Autodesk Inventor part; units mm, degrees
ref_plane "YZ Plane" through (0, 0, 0) normal (1, 0, 0) x (0, 1, 0)
ref_plane "XZ Plane" through (0, 0, 0) normal (0, 1, 0) x (-1, 0, 0)
ref_plane "XY Plane" through (0, 0, 0) normal (0, 0, 1) x (1, 0, 0)
sketch "Sketch1" plane through (0, 0, 0) normal (0, 0, 1) x (1, 0, 0)
  line L0 (-7.5, 17.5) -> (7.5, 17.5)
  line L1 (7.5, 17.5) -> (7.5, -17.5)
  line L2 (7.5, -17.5) -> (-7.5, -17.5)
  line L3 (-7.5, -17.5) -> (-7.5, 17.5)
  line L4 (-7.5, 17.5) -> (7.5, -17.5) construction
  line L5 (7.5, 17.5) -> (-7.5, -17.5) construction
  point P0 (0, 0)
  dimension "d0" = 15
  dimension "d1" = 35
extrude "Extrusion1" add sketch "Sketch1" along normal blind 25
sketch "Sketch2" plane through (-7.5, 17.5, 0) normal (0, 1, 0) x (1, 0, 0)
  line L0 (15, -25) -> (0, -25) construction
  line L1 (0, 0) -> (10.4, 0) construction
  line L2 (10.4, 0) -> (10.4, -25) construction
  line L3 (10.4, -25) -> (0, -25) construction
  line L4 (0, -25) -> (0, 0) construction
  line L5 (0, 0) -> (15, 0) construction
  line L6 (5.2, 0) -> (5.2, -25) construction
  line L7 (10.4, -12.5) -> (0, -12.5) construction
  line L8 (0, 0) -> (0, -25) construction
  line L9 (10.4, -4.3) -> (0, -4.3) construction
  line L10 (0, -4.3) -> (0, -20.7) construction
  line L11 (0, -20.7) -> (10.4, -20.7) construction
  line L12 (10.4, -20.7) -> (10.4, -4.3) construction
  line L13 (10.4, -4.3) -> (0, -20.7) construction
  line L14 (0, -4.3) -> (10.4, -20.7) construction
  circle A0 centre (5.2, -9.5) radius 5.2
  circle A1 centre (5.2, -15.5) radius 5.2
  line L15 (10.4, -9.5) -> (0, -9.5)
  line L16 (0, -9.5) -> (0, -15.5)
  line L17 (0, -15.5) -> (10.4, -15.5)
  line L18 (10.4, -15.5) -> (10.4, -9.5)
  line L19 (10.4, -9.5) -> (0, -15.5) construction
  line L20 (0, -9.5) -> (10.4, -15.5) construction
  point P0 (7.5, 0)
  point P1 (5.2, -12.5)
  dimension "d4" = 10.4
  dimension "d5" = 16.4
extrude "Extrusion2" cut sketch "Sketch2" against normal blind 35
sketch "Sketch3" plane through (-7.5, -17.5, 0) normal (-1, 0, 0) x (0, 0, 1)
  line L0 (25, 35) -> (25, 0)
  line L1 (0, 0) -> (0, 35)
  line L2 (25, 13.0367) -> (0, 13.0367)
  line L3 (0, 13.0367) -> (0, 12.8367)
  line L4 (0, 12.8367) -> (25, 12.8367)
  line L5 (25, 12.8367) -> (25, 13.0367)
  point P0 (0, 17.5)
  dimension "d8" = 0.2
extrude "Extrusion3" cut sketch "Sketch3" against normal blind 11
properties part number "Cutting Tool V1"
Geometry check sheet. Reference: the model listing, model coordinates, mm. A direction names the side the tool comes from. Round coordinates to 2 decimals unless told otherwise and drop trailing zeros. Loops run counter-clockwise (first coordinate to the right, second up) from the corner with the lowest first, then second, coordinate; pieces in that order, holes last. Notation, with made-up numbers: (89, 44) - (142, 44) arc R23 ccw to (142, 68) - close; hole circle Ø6 at (48.25, -5.5). An arc over 180 degrees is marked (long way). One line per question, with ' | ' between items. Start each with the question number.
1. Tool access check on faces 1 (the face through (3, -4.663, 7)), 2 (the face through (2.9, -11, 13)), 3 (the face through (-2.4, 6.7, 20.7)), 4 (the face through (0, 0, 25)). Record the directions out of +Z, -Z, +X, -X, +Y, -Y that give a thin tool (end or side, any length) a straight path to the whole face; none if there is none.
2. Cross-section at D-D on y = -4. Record the cut outline in (x, z), then the cut area to 3 significant figures.
3. Depth check by flat-ended pin: pin 1 (5.5 mm diameter, centred on x = -1, z = 14, fed in from -Y); pin 2 (3 mm diameter, centred on y = 9.5, z = 11.5, fed in from -X). Enter the tip coordinate at first touch or a pass-through.
4. Cross-section at A-A on z = 8.5. Record the cut outline in (x, y).
5. Cross-section at B-B on x = -2.3. Record the cut outline in (y, z), then the cut area to 3 significant figures.
6. Scan lines: line 1 (Y direction, x = -1.25, z = 3.75); line 2 (X direction, y = -4, z = 5.5); line 3 (X direction, y = 14.5, z = 13.5). Record each from-to range of solid material in increasing order. Write a range as [from, to].
7. Cross-section at C-C on z = 13.25. Record the cut outline in (x, y), then the cut area to 3 significant figures.
8. Draft check along Z on faces 5 (the face through (3, -4.463, 18)), 6 (the face through (-2.4, -11, 20.7)), 7 (the face through (0, 0, 0)). Enter one of: released by +Z, released by -Z, zero draft, split by the parting line, or undercut.
Taken from the geometry:
1) face 1: +Z, -Z, -X | face 2: -X, +Y, -Y | face 3: +Y, -Y | face 4: +Z, +X, -X, +Y, -Y
2) outline: (-7.5, 0) - (7.5, 0) - (7.5, 25) - (-7.5, 25) - (-7.5, 15.5) arc R5.2 cw to (2.9, 15.5) - (2.9, 9.5) arc R5.2 cw to (-7.5, 9.5) - close | area: 228 mm²
3) pin 1: through | pin 2: x = 2.9
4) outline: (-7.5, -17.5) - (-7.4, -17.5) - (-7.4, -4.66) - (-7.5, -4.66) - close; (-7.5, -4.46) - (-7.4, -4.46) - (-7.4, 17.5) - (-7.5, 17.5) - close; (2.8, -17.5) - (7.5, -17.5) - (7.5, 17.5) - (2.8, 17.5) - (2.8, -4.46) - (3.5, -4.46) - (3.5, -4.66) - (2.8, -4.66) - close
5) outline: (-17.5, 0) - (-4.66, 0) - (-4.66, 4.3) - (-17.5, 4.3) - close; (-17.5, 20.7) - (-4.66, 20.7) - (-4.66, 25) - (-17.5, 25) - close; (-4.46, 0) - (17.5, 0) - (17.5, 4.3) - (-4.46, 4.3) - close; (-4.46, 20.7) - (17.5, 20.7) - (17.5, 25) - (-4.46, 25) - close | area: 299 mm²
6) line 1: [-17.5, -4.66], [-4.46, 17.5] | line 2: [-7.5, -5.62], [1.02, 7.5] | line 3: [2.9, 7.5]
7) outline: (2.9, -17.5) - (7.5, -17.5) - (7.5, 17.5) - (2.9, 17.5) - (2.9, -4.46) - (3.5, -4.46) - (3.5, -4.66) - (2.9, -4.66) - close | area: 161 mm²
8) face 5: zero draft | face 6: undercut | face 7: released by -Z
